Here's how the part is built. I have some questions about the finished solid (model axes, mm). Face numbers are marked on the shaded views. A direction names the side the tool comes from. Coordinates: 2 decimals unless noted, no trailing zeros. Write each loop counter-clockwise with the first axis right and the second up, starting at its lowest first coordinate (ties: lowest second). Pieces come first, ordered by that corner, then holes. Notation, with made-up numbers: (76, 87.25) -> (129, 87.25) arc R19 ccw to (129, 109.25) -> close; hole circle Ø11 at (33.5, 66.25). An arc over 180 degrees is marked (long way). Put each result on its own line as item: value. Start each with the question number.
Item 1: I need wall thicknesses on line 1 (Z direction, x = 7, y = 21); line 2 (Y direction, x = -7.5, z = -2); line 3 (Y direction, x = 3, z = -5). Which ranges of each line are inside material? Lowest first, please. Write a range as [from, to].
Item 2: I want a section at C-C, the plane y = -25.5. List the corners of the cut face in (x, z) for me.
Item 3: I want a section at D-D, the plane x = 10.5. List the corners of the cut face in (y, z) for me, then the cut area to 3 significant figures.
Item 4: I want a section at A-A, the plane z = 0. List the corners of the cut face in (x, y) for me, then the cut area to 4 significant figures.
Item 5: For pin 1 (1 mm diameter, centred on y = 22, z = -9.5, fed in from +X); pin 2 (2 mm diameter, centred on x = -7.5, y = 16, fed in from +Z); pin 3 (3.5 mm diameter, centred on x = 8.5, z = -14, fed in from +Y); pin 4 (18.5 mm diameter, centred on x = 4.5, z = -1.5, fed in from +Y), each with a flat end and sliding along its axis, tell me the tip position at first contact or that it passes through.
Item 6: On a 3-axis mill with a long thin cutter (end or side, diameter ignored), from which of +Z, -Z, +X, -X, +Y, -Y can I reach the whole of each face in a straight line? I mean the marked faces 1, 2 and 3. Say none if no direction works.
Item 7: I want a section at B-B, the plane x = 0. List the corners of the cut face in (y, z) for me, then the cut area to 3 significant figures.
from build123d import *

# Parameters (mm, degrees)
SKETCH_1_R          = 16.5
EXTRUDE_1_DEPTH     = 33
SKETCH_1_3_R        = 18.5
EXTRUDE_2_DEPTH     = 23
SKETCH_3_R          = 1.5
CUT_EXTRUDE_1_DEPTH = 2.5
SKETCH_3_3_R        = 3
EXTRUDE_3_DEPTH     = 18
SKETCH_3_4_R        = 6
EXTRUDE_4_DEPTH     = 6
CUT_EXTRUDE_START   = -12
CUT_EXTRUDE_2_DEPTH = 12


with BuildPart() as part:
    # Sketch 1 → Extrude 1 (new body)
    with BuildSketch(Plane(origin=(0, 0, 0), x_dir=(1, 0, 0), z_dir=(0, 1, 0))):
        with Locations(Location((0, 0, 0), (0, 0, 270))):
            Circle(SKETCH_1_R)
    extrude(amount=-EXTRUDE_1_DEPTH)

    # Sketch 1_3 → Extrude 2 (add)
    with BuildSketch(Plane(origin=(0, 0, 0), x_dir=(1, 0, 0), z_dir=(0, 1, 0))):
        with Locations(Location((0, 0, 0), (0, 0, 270))):
            Circle(SKETCH_1_3_R)
    extrude(amount=EXTRUDE_2_DEPTH)

    # Sketch 3 → Cut-Extrude 1 (cut)
    with BuildSketch(Plane(origin=(0, 23, 0), x_dir=(1, 0, 0), z_dir=(0, 1, 0))):
        with Locations(Location((-7.75, 13.423393759, 0), (0, 0, 270))):
            Circle(SKETCH_3_R)
        with Locations(Location((7.75, 13.423393759, 0), (0, 0, 270))):
            Circle(SKETCH_3_R)
        with Locations(Location((15.5, 0, 0), (0, 0, 270))):
            Circle(SKETCH_3_R)
        with Locations(Location((7.75, -13.423393759, 0), (0, 0, 270))):
            Circle(SKETCH_3_R)
        with Locations(Location((-7.75, -13.423393759, 0), (0, 0, 270))):
            Circle(SKETCH_3_R)
        with Locations(Location((-15.5, 0, 0), (0, 0, 270))):
            Circle(SKETCH_3_R)
    extrude(amount=-CUT_EXTRUDE_1_DEPTH, mode=Mode.SUBTRACT)

    # Sketch 3_3 → Extrude 3 (add)
    with BuildSketch(Plane(origin=(0, 23, 0), x_dir=(1, 0, 0), z_dir=(0, 1, 0))):
        with Locations(Location((0, 7, 0), (0, 0, 270))):
            Circle(SKETCH_3_3_R)
    extrude(amount=EXTRUDE_3_DEPTH)

    # Sketch 3_4 → Extrude 4 (add)
    with BuildSketch(Plane(origin=(0, 23, 0), x_dir=(1, 0, 0), z_dir=(0, 1, 0))):
        with Locations(Location((0, 7, 0), (0, 0, 270))):
            Circle(SKETCH_3_4_R)
    extrude(amount=EXTRUDE_4_DEPTH)

    # Sketch 4 → Cut-Extrude 2 (cut)
    with BuildSketch(Plane(origin=(0, 41, 0), x_dir=(1, 0, 0), z_dir=(0, 1, 0)).offset(CUT_EXTRUDE_START)):
        with BuildLine():
            Line((-1.658312395, 9.5), (1.658312395, 9.5))
            ThreePointArc((1.658312395, 9.5), (0, 10), (-1.658312395, 9.5))
        make_face()
    extrude(amount=CUT_EXTRUDE_2_DEPTH, mode=Mode.SUBTRACT)


solid = part.part
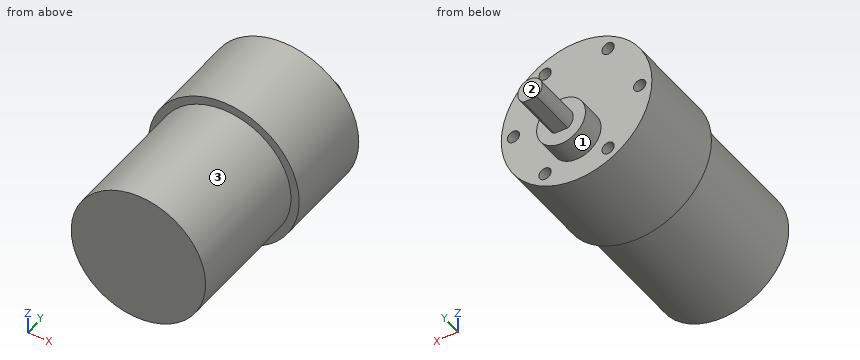
Calculated:
1. line 1: z = [-17.12, -14.72], [-12.12, 12.12], [14.72, 17.12]
1. line 2: y = [-33, 23]
1. line 3: y = [-33, 29]
2. outline: circle Ø33 at (0, 0)
3. outline: (-33, -12.73) -> (0, -12.73) -> (0, -15.23) -> (23, -15.23) -> (23, 15.23) -> (0, 15.23) -> (0, 12.73) -> (-33, 12.73) -> close
3. area: 1,540 mm2
4. outline: (-18.5, 0) -> (-16.5, 0) -> (-16.5, -33) -> (16.5, -33) -> (16.5, 0) -> (18.5, 0) -> (18.5, 23) -> (17, 23) -> (17, 20.5) -> (14, 20.5) -> (14, 23) -> (-14, 23) -> (-14, 20.5) -> (-17, 20.5) -> (-17, 23) -> (-18.5, 23) -> close
4. area: 1,925 mm2
5. pin 1: stops at x = 16.16
5. pin 2: stops at z = 17.32
5. pin 3: stops at y = 23
5. pin 4: stops at y = 41
6. face 1: +Y
6. face 2: +Z, -Z, +X, -X, +Y
6. face 3: -Y
7. outline: (-33, -16.5) -> (0, -16.5) -> (0, -18.5) -> (23, -18.5) -> (23, -13) -> (29, -13) -> (29, -9.5) -> (41, -9.5) -> (41, -4) -> (29, -4) -> (29, -1) -> (23, -1) -> (23, 18.5) -> (0, 18.5) -> (0, 16.5) -> (-33, 16.5) -> close
7. area: 2,080 mm2
